from build123d import *

# Parameters (mm, degrees)
SKETCH1_W                    = 25.4
SKETCH1_H                    = 25.4
BOSS_EXTRUDE1_DEPTH          = 25.4
SKETCH2_R                    = 2.25
CUT_EXTRUDE1_DEPTH           = 12.7
SKETCH3_R                    = 6.985
CUT_EXTRUDE2_DEPTH           = 12.7
F_6_32_TAPPED_HOLE1_REACH    = 33.109
F_6_32_TAPPED_HOLE1_BORE_R   = 1.35255
F_1_4_20_TAPPED_HOLE2_REACH  = 33.109
F_1_4_20_TAPPED_HOLE2_BORE_R = 2.5527


with BuildPart() as part:
    # Sketch1 → Boss-Extrude1 (new body)
    with BuildSketch(Plane(origin=(0, 0, 0), x_dir=(1, 0, 0), z_dir=(0, 1, 0))):
        Rectangle(SKETCH1_W, SKETCH1_H)
    extrude(amount=BOSS_EXTRUDE1_DEPTH)

    # Sketch2 → Cut-Extrude1 (cut)
    with BuildSketch(Plane.XY.offset(12.7)):
        with Locations((0, 12.7)):
            Circle(SKETCH2_R)
    extrude(amount=-CUT_EXTRUDE1_DEPTH, mode=Mode.SUBTRACT)

    # Sketch3 → Cut-Extrude2 (cut)
    with BuildSketch(Plane(origin=(0, 0, -12.7), x_dir=(-1, 0, 0), z_dir=(0, 0, -1))):
        with Locations((0, 12.7)):
            Circle(SKETCH3_R)
    extrude(amount=-CUT_EXTRUDE2_DEPTH, mode=Mode.SUBTRACT)

    # #6-32 Tapped Hole1 bore → #6-32 Tapped Hole1 (cut, up to next)
    with BuildSketch(Plane(origin=(0, 25.4, 0), x_dir=(1, 0, 0), z_dir=(0, 1, 0)), mode=Mode.PRIVATE) as f_6_32_tapped_hole1_sk1:
        with Locations((0, -6.35)):
            Circle(F_6_32_TAPPED_HOLE1_BORE_R)
    f_6_32_tapped_hole1_tool1 = extrude(f_6_32_tapped_hole1_sk1.sketch, amount=-F_6_32_TAPPED_HOLE1_REACH, mode=Mode.PRIVATE) & part.part
    add(f_6_32_tapped_hole1_tool1.solids().sort_by_distance((0, 25.4, 6.35))[0], mode=Mode.SUBTRACT)

    # 1/4-20 Tapped Hole2 bore → 1/4-20 Tapped Hole2 (cut, up to next)
    with BuildSketch(Plane(origin=(0, 25.4, 0), x_dir=(1, 0, 0), z_dir=(0, 1, 0)), mode=Mode.PRIVATE) as f_1_4_20_tapped_hole2_sk1:
        with Locations((0, 6.35)):
            Circle(F_1_4_20_TAPPED_HOLE2_BORE_R)
    f_1_4_20_tapped_hole2_tool1 = extrude(f_1_4_20_tapped_hole2_sk1.sketch, amount=-F_1_4_20_TAPPED_HOLE2_REACH, mode=Mode.PRIVATE) & part.part
    add(f_1_4_20_tapped_hole2_tool1.solids().sort_by_distance((0, 25.4, -6.35))[0], mode=Mode.SUBTRACT)


solid = part.part
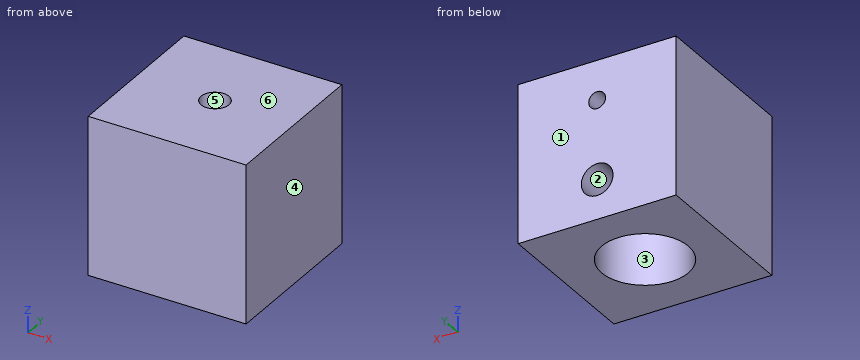
Geometry check sheet. Reference: the model listing, model coordinates, mm. Face numbers are marked on the shaded views. A direction names the side the tool comes from. Round coordinates to 2 decimals unless told otherwise and drop trailing zeros. Loops run counter-clockwise (first coordinate to the right, second up) from the corner with the lowest first, then second, coordinate; pieces in that order, holes last. Notation, with made-up numbers: (1.5, 46) - (50.5, 46) arc R13 ccw to (50.5, 67) - close; hole circle Ø2 at (89.5, 21.5). An arc over 180 degrees is marked (long way). Answer as CSV lines item,"result".
(1) Material ranges on line 1 along X through (y, z) = (22, 6.35); line 2 along Z through (x, y) = (0, 23.75); line 3 along X through (y, z) = (23, -6.35), recorded low to high.
Output values:
line 1,"x = -12.7 to -1.35, 1.35 to 12.7"
line 2,"z = -12.7 to -8.9, -3.8 to 5, 7.7 to 12.7"
line 3,"x = -12.7 to -2.55, 2.55 to 12.7"
(2) Cross-section at A-A, the plane y = 12.7. Enter the section's corners in (x, z) (3 decimals).
Output values:
outline,"(-12.7, -12.7) - (-6.985, -12.7) - (-6.985, 0) - (-2.25, 0) - (-2.25, 12.7) - (-12.7, 12.7) - close; (2.25, 0) - (6.985, 0) - (6.985, -12.7) - (12.7, -12.7) - (12.7, 12.7) - (2.25, 12.7) - close"
(3) Release check for a two-part mould opening along X. For the marked faces 4, 5 and 6 record: released by +X, released by -X, zero draft, split by the parting line, or undercut.
Output values:
face 4,"released by +X"
face 5,"undercut"
face 6,"zero draft"
(4) Set-up check for the marked faces 1, 2 and 3: record each of +Z, -Z, +X, -X, +Y, -Y from which the full face is reachable in a straight line by a thin tool's end or side.
Output values:
face 1,"+Z, -Z, +X, -X, +Y"
face 2,"+Y"
face 3,"-Z"
(5) Depth check by flat-ended pin: pin 1 Ø4 at (x, y) = (-3, 15.5) entering from -Z; pin 2 Ø1.6 at (x, z) = (0, 6.35) entering from +Y. Enter the tip coordinate at first touch or a pass-through.
Output values:
pin 1,"stops at z = 0"
pin 2,"stops at y = 10.6"
(6) Cross-section at C-C, the plane z = 6.35. Enter the section's corners in (x, y).
Output values:
outline,"(-12.7, 0) - (12.7, 0) - (12.7, 25.4) - (1.35, 25.4) - (1.35, 14.5) arc R2.25 cw (long way) to (-1.35, 14.5) - (-1.35, 25.4) - (-12.7, 25.4) - close"
(7) Cross-section at B-B, the plane x = 0. Enter the section's corners in (y, z) (3 decimals).
Output values:
outline,"(0, -12.7) - (5.715, -12.7) - (5.715, 0) - (10.45, 0) - (10.45, 12.7) - (0, 12.7) - close; (14.95, 0) - (19.685, 0) - (19.685, -3.797) - (25.4, -3.797) - (25.4, 4.997) - (14.95, 4.997) - close; (14.95, 7.703) - (25.4, 7.703) - (25.4, 12.7) - (14.95, 12.7) - close; (19.685, -12.7) - (25.4, -12.7) - (25.4, -8.903) - (19.685, -8.903) - close"
(8) Cross-section at D-D, the plane y = 23.5. Enter the section's corners in (x, z), and give its area (3 significant figures).
Output values:
outline,"(-12.7, -12.7) - (12.7, -12.7) - (12.7, 12.7) - (-12.7, 12.7) - close; hole circle Ø5.11 at (0, -6.35); hole circle Ø2.71 at (0, 6.35)"
area,"619 mm²"
